Geometry: see drawing. Coordinates: mm, zero at the bounding-box minimum. A direction names the side the tool comes from. Coordinates: 2 decimals unless noted, no trailing zeros. Loops run counter-clockwise (first coordinate to the right, second up) from the corner with the lowest first, then second, coordinate; pieces in that order, holes last.
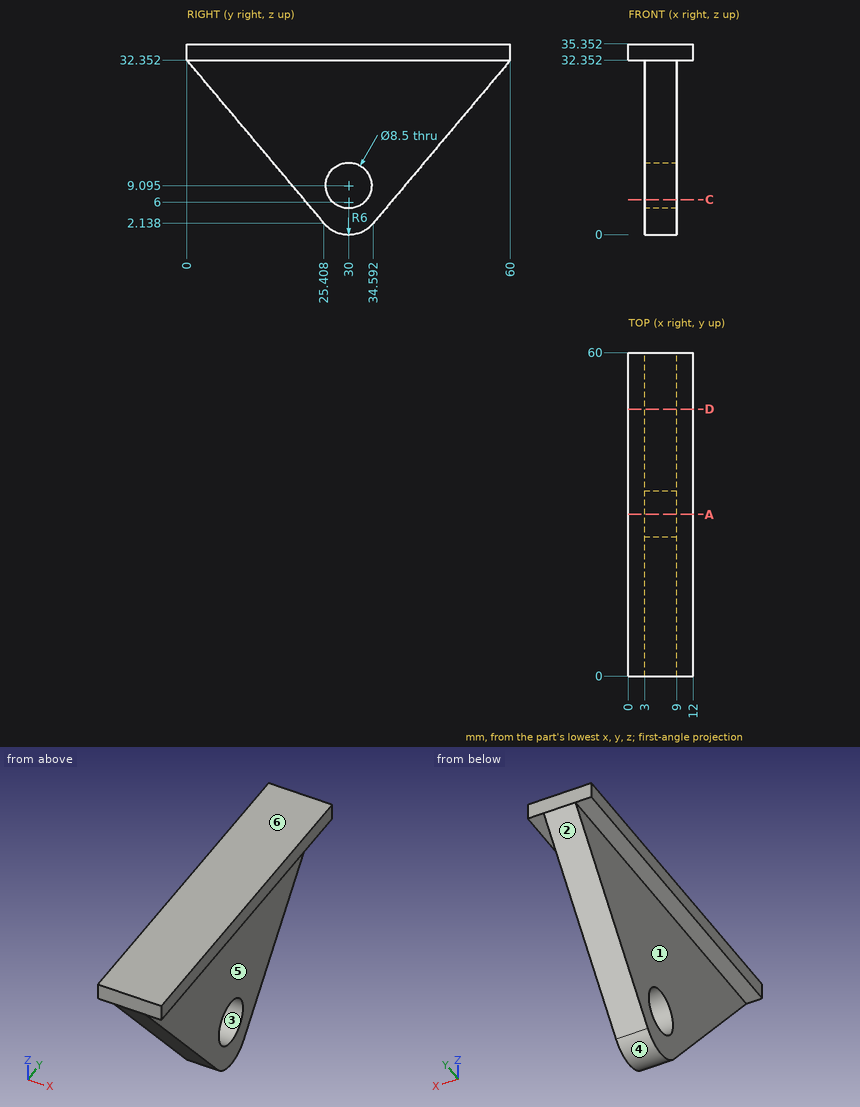
Item 1: Section query A-A (y = 30). Output: boundary loops of the cut face in (x, z) (1 decimal).
Result:
outline: (0, 32.4) - (3, 32.4) - (3, 13.3) - (9, 13.3) - (9, 32.4) - (12, 32.4) - (12, 35.4) - (0, 35.4) - close; (3, 0) - (9, 0) - (9, 4.8) - (3, 4.8) - close
Item 2: Mould query, pull axis Y, two halves, no side actions, for the marked faces 1, 2, 3 and 4. Classes: +Y half, -Y half, draft (parallel to the pull), parting line (faces both ways), or undercut.
Result:
face 1: draft
face 2: +Y half
face 3: undercut
face 4: parting line
Item 3: Contact query for flat-ended pins moving along their axis: P1, Ø6, axis at x = 9, y = 49, coming from the -Z side (1 decimal); P2, Ø6, axis at x = 8, y = 7.5, coming from the -Z side (1 decimal); P3, Ø2, axis at x = 3.5, y = 9, coming from the -Z side; P4, Ø5, axis at y = 30, z = 9.09, coming from the -X side. Output: stop coordinate, or through.
Result:
P1: stops at z = 15.7
P2: stops at z = 19.9
P3: stops at z = 20.46
P4: passes through
Item 4: Section query D-D (y = 49.5). Output: boundary loops of the cut face in (x, z).
Result:
outline: (0, 32.35) - (3, 32.35) - (3, 19.87) - (9, 19.87) - (9, 32.35) - (12, 32.35) - (12, 35.35) - (0, 35.35) - close
Item 5: Reachability of the marked faces 5 and 6 from +Z, -Z, +X, -X, +Y, -Y: full face, straight path, thin tool, end or side. Return the list, or none.
Result:
face 5: -Z, +X, +Y, -Y
face 6: +Z, +X, -X, +Y, -Y
Item 6: Section query C-C (z = 6.5). Output: boundary loops of the cut face in (x, y).
Result:
outline: (3, 21.74) - (9, 21.74) - (9, 26.63) - (3, 26.63) - close; (3, 33.37) - (9, 33.37) - (9, 38.26) - (3, 38.26) - close
Item 7: Line query: L1, parallel to Z at x = 1, y = 46.5; L2, parallel to X at y = 30.5, z = 17; L3, parallel to Y at x = 6, z = 10 (1 decimal). Output: solid intervals per line, ascending.
Result:
L1: z = 32.35 to 35.35
L2: x = 3 to 9
L3: y = 18.8 to 25.8, 34.2 to 41.2
